from build123d import *

# Parameters (mm, degrees)
SKETCH1_R           = 2.38125
BOSS_EXTRUDE1_DEPTH = 203.2


with BuildPart() as part:
    # Sketch1 → Boss-Extrude1 (new body)
    with BuildSketch(Plane(origin=(0, 0, 0), x_dir=(0, 0, -1), z_dir=(1, 0, 0))):
        with BuildLine():
            Line((7.039054482, 0.508), (3.959468146, 5.842))
            ThreePointArc((3.959468146, 5.842), (3.587586336, 6.21388181), (3.079586336, 6.35))
            Line((3.079586336, 6.35), (-3.079586336, 6.35))
            ThreePointArc((-3.079586336, 6.35), (-3.587586336, 6.21388181), (-3.959468146, 5.842))
            Line((-3.959468146, 5.842), (-7.039054482, 0.508))
            ThreePointArc((-7.039054482, 0.508), (-7.175172672, 0), (-7.039054482, -0.508))
            Line((-7.039054482, -0.508), (-3.959468146, -5.842))
            ThreePointArc((-3.959468146, -5.842), (-3.587586336, -6.21388181), (-3.079586336, -6.35))
            Line((-3.079586336, -6.35), (3.079586336, -6.35))
            ThreePointArc((3.079586336, -6.35), (3.587586336, -6.21388181), (3.959468146, -5.842))
            Line((3.959468146, -5.842), (7.039054482, -0.508))
            ThreePointArc((7.039054482, -0.508), (7.175172672, 0), (7.039054482, 0.508))
        make_face()
        Circle(SKETCH1_R, mode=Mode.SUBTRACT)
    extrude(amount=BOSS_EXTRUDE1_DEPTH)


solid = part.part
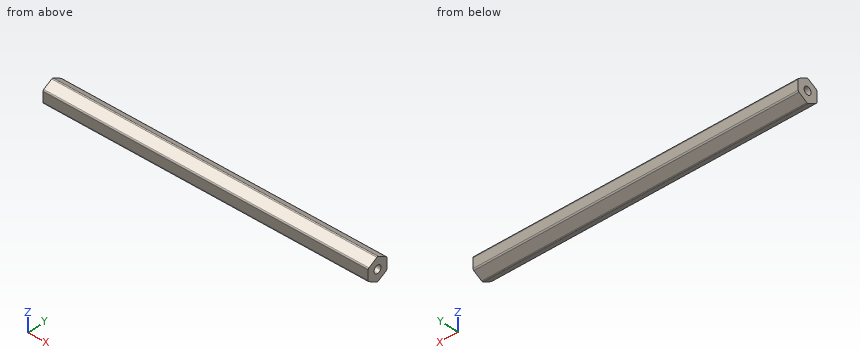
Part model, mm, in its own coordinate system. Give positions to 0.01 mm unless a question says otherwise; leave off trailing zeros. Write each loop counter-clockwise with the first axis right and the second up, starting at its lowest first coordinate (ties: lowest second). Pieces come first, ordered by that corner, then holes.
1) Cut at B-B on x = 138.5. Write the cut outline in (y, z), then the cut area to 3 significant figures.
Resolved:
outline: (-6.35, -3.08) arc R1.02 ccw to (-5.84, -3.96) - (-0.51, -7.04) arc R1.02 ccw to (0.51, -7.04) - (5.84, -3.96) arc R1.02 ccw to (6.35, -3.08) - (6.35, 3.08) arc R1.02 ccw to (5.84, 3.96) - (0.51, 7.04) arc R1.02 ccw to (-0.51, 7.04) - (-5.84, 3.96) arc R1.02 ccw to (-6.35, 3.08) - close; hole circle Ø4.76 at (0, 0)
area: 122 mm2
2) Probe L1, parallel to Y at x = 116, z = -0.25; L2, parallel to Z at x = 164.5, y = -0.75; L3, parallel to Z at x = 30.5, y = 0.5. List the from-to ranges inside material, lowest first.
Resolved:
L1: y = -6.35 to -2.37, 2.37 to 6.35
L2: z = -6.9 to -2.26, 2.26 to 6.9
L3: z = -7.04 to -2.33, 2.33 to 7.04
3) Cut at A-A on z = 0. Write the cut outline in (x, y), then the cut area to 3 significant figures.
Resolved:
outline: (0, -6.35) - (203.2, -6.35) - (203.2, -2.38) - (0, -2.38) - close; (0, 2.38) - (203.2, 2.38) - (203.2, 6.35) - (0, 6.35) - close
area: 1,610 mm2
4) Pin check, flat tips, straight feed: pin 1 (2 mm diameter, centred on x = 100, y = 2, fed in from -Z) (3 decimals); pin 2 (4 mm diameter, centred on x = 170.5, y = -3.5, fed in from -Z); pin 3 (2 mm diameter, centred on x = 129.5, z = -5.5, fed in from +Y). Stop position of each tip, or through.
Resolved:
pin 1: stops at z = -6.755
pin 2: stops at z = -6.47
pin 3: stops at y = 4.91
